Autodesk Inventor part; units mm, degrees
ref_plane "YZ Plane" through (0, 0, 0) normal (1, 0, 0) x (0, 1, 0)
ref_plane "XZ Plane" through (0, 0, 0) normal (0, 1, 0) x (-1, 0, 0)
ref_plane "XY Plane" through (0, 0, 0) normal (0, 0, 1) x (1, 0, 0)
sketch "スケッチ1" plane through (0, 0, 0) normal (0, 0, 1) x (1, 0, 0)
  line L0 (-10, -7) -> (-5, -7)
  line L1 (10, -7) -> (10, 0)
  line L2 (10, 0) -> (-10, 0)
  line L3 (-10, 0) -> (-10, -7)
  line L4 (-10, -7) -> (10, 0) construction
  line L5 (10, -7) -> (-10, 0) construction
  line L6 (-5, -2.5) -> (5, -2.5)
  line L7 (5, -2.5) -> (5, -7)
  line L8 (-5, -7) -> (-5, -2.5)
  line L9 (-5, -2.5) -> (5, -7) construction
  line L10 (5, -2.5) -> (-5, -7) construction
  line L11 (5, -7) -> (10, -7)
  point P0 (0, 0)
  point P1 (0, -3.5)
  point P2 (0, -4.75)
  dimension "d0" = 20
  dimension "d1" = 7
  dimension "d2" = 10
  dimension "d3" = 4.5
extrude "押し出し1" add sketch "スケッチ1" along normal blind 30
sketch "スケッチ2" plane through (-10, 0, 0) normal (0, 1, 0) x (1, 0, 0)
  line L0 (0, 0) -> (0, -30)
  line L1 (20, 0) -> (0, 0)
  line L2 (20, -30) -> (0, -30)
  line L3 (20, 0) -> (20, -30)
  point P0 (10, 0)
  point P1 (3.5, -8.5)
  point P2 (3.5, -21.5)
  point P3 (16.5, -21.5)
  point P4 (16.5, -8.5)
  dimension "d6" = 3.5
  dimension "d7" = 3.5
  dimension "d8" = 8.5
  dimension "d9" = 8.5
  dimension "d10" = 3.5
  dimension "d11" = 3.5
  dimension "d12" = 8.5
  dimension "d13" = 8.5
hole "穴1" at (-6.5, 0, 8.5) at (-6.5, 0, 21.5) at (6.5, 0, 21.5) at (6.5, 0, 8.5) direction (0, -1, 0) diameter 3 end through all
properties part number "slider_b7p5x20_30_sa" material "アルミニウム 6061-AHC"
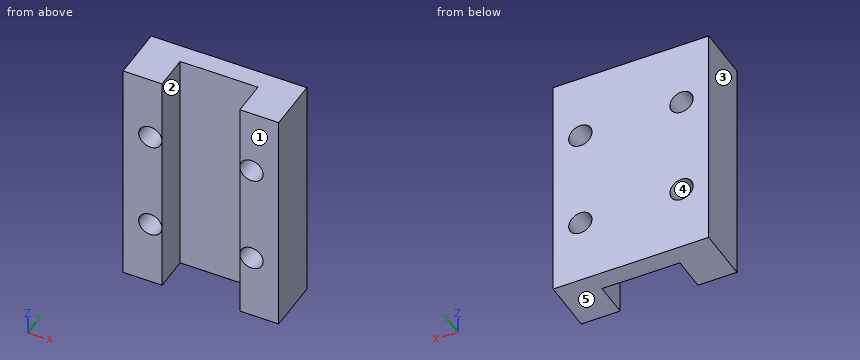
Read the model definition and answer for the solid it produces. Units are mm, in the model's axes. Face numbers are marked on the shaded views. A direction names the side the tool comes from. Coordinates: 2 decimals unless noted, no trailing zeros. Loops run counter-clockwise (first coordinate to the right, second up) from the corner with the lowest first, then second, coordinate; pieces in that order, holes last. Notation, with made-up numbers: (34.25, 83.5) - (73.25, 83.5) arc R5 ccw to (73.25, 89.5) - close; hole circle Ø5 at (5, 36.5). An arc over 180 degrees is marked (long way). Answer in a Markdown table with one row per item.
Q1. Find section C-C on z = 27.5. Write down the section's boundary in (x, y).
Here are the results:
| item | result |
|---|---|
| outline | (-10, -7) - (-5, -7) - (-5, -2.5) - (5, -2.5) - (5, -7) - (10, -7) - (10, 0) - (-10, 0) - close |
Q2. Find section D-D on z = 7.5. Write down the section's boundary in (x, y), plus the area to 3 significant figures.
Here are the results:
| item | result |
|---|---|
| outline | (-10, -7) - (-7.62, -7) - (-7.62, 0) - (-10, 0) - close; (-5.38, -7) - (-5, -7) - (-5, -2.5) - (5, -2.5) - (5, -7) - (5.38, -7) - (5.38, 0) - (-5.38, 0) - close; (7.62, -7) - (10, -7) - (10, 0) - (7.62, 0) - close |
| area | 63.7 mm^2 |
Q3. Find section A-A on y = -1.25. Write down the section's boundary in (x, z).
Here are the results:
| item | result |
|---|---|
| outline | (-10, 0) - (10, 0) - (10, 30) - (-10, 30) - close; hole circle Ø3 at (-6.5, 8.5); hole circle Ø3 at (-6.5, 21.5); hole circle Ø3 at (6.5, 8.5); hole circle Ø3 at (6.5, 21.5) |
Q4. For the marked faces 1 and 2, determine the directions among +Z, -Z, +X, -X, +Y, -Y from which every point of the face is accessible in a straight line to the end or side of a thin tool.
Here are the results:
| item | result |
|---|---|
| face 1 | +Z, -Z, +X, -X, -Y |
| face 2 | +Z, -Z, -Y |
Q5. The mould has two halves that part along X. Classify the marked faces 3, 4 and 5: pulls with the +X half, pulls with the -X half, needs draft (parallel to the pull), parting line crosses it, or undercut.
Here are the results:
| item | result |
|---|---|
| face 3 | pulls with the -X half |
| face 4 | undercut |
| face 5 | needs draft |
Q6. Given P1, Ø2.5, axis at x = -6.5, z = 8.5, coming from the +Y side; P2, Ø3, axis at x = -2.5, z = 10, coming from the -Y side, each flat-ended and moving along its own axis, determine where each tip first touches the part or whether it passes through.
Here are the results:
| item | result |
|---|---|
| P1 | passes through |
| P2 | stops at y = -2.5 |
Q7. Find section B-B on x = 6.5. Write down the section's boundary in (y, z), plus the area to 3 significant figures.
Here are the results:
| item | result |
|---|---|
| outline | (-7, 0) - (0, 0) - (0, 7) - (-7, 7) - close; (-7, 10) - (0, 10) - (0, 20) - (-7, 20) - close; (-7, 23) - (0, 23) - (0, 30) - (-7, 30) - close |
| area | 168 mm^2 |
Q8. Straight lines are drawn through the part: line 1 along Z through (x, y) = (-6.5, -2); line 2 along X through (y, z) = (-2, 21.5); line 3 along X through (y, z) = (-5.25, 24.75). For each, find the intervals that lie inside material, in ascending order. Write a range as [from, to].
Here are the results:
| item | result |
|---|---|
| line 1 | z = [0, 7], [10, 20], [23, 30] |
| line 2 | x = [-10, -8], [-5, 5], [8, 10] |
| line 3 | x = [-10, -5], [5, 10] |
